Answer from the drawing. Dimensions are ordinates in mm from the lowest x, y and z of the part. A direction names the side the tool comes from. Give positions to 0.01 mm unless a question says otherwise; leave off trailing zeros. Write each loop counter-clockwise with the first axis right and the second up, starting at its lowest first coordinate (ties: lowest second). Pieces come first, ordered by that corner, then holes. Notation, with made-up numbers: M 26,18.25 L 66,18.25 A23 ccw 66,39.25 Z; hole C -26,57.25 d1. An arc over 180 degrees is marked long. Put each result on its own line as item: value.
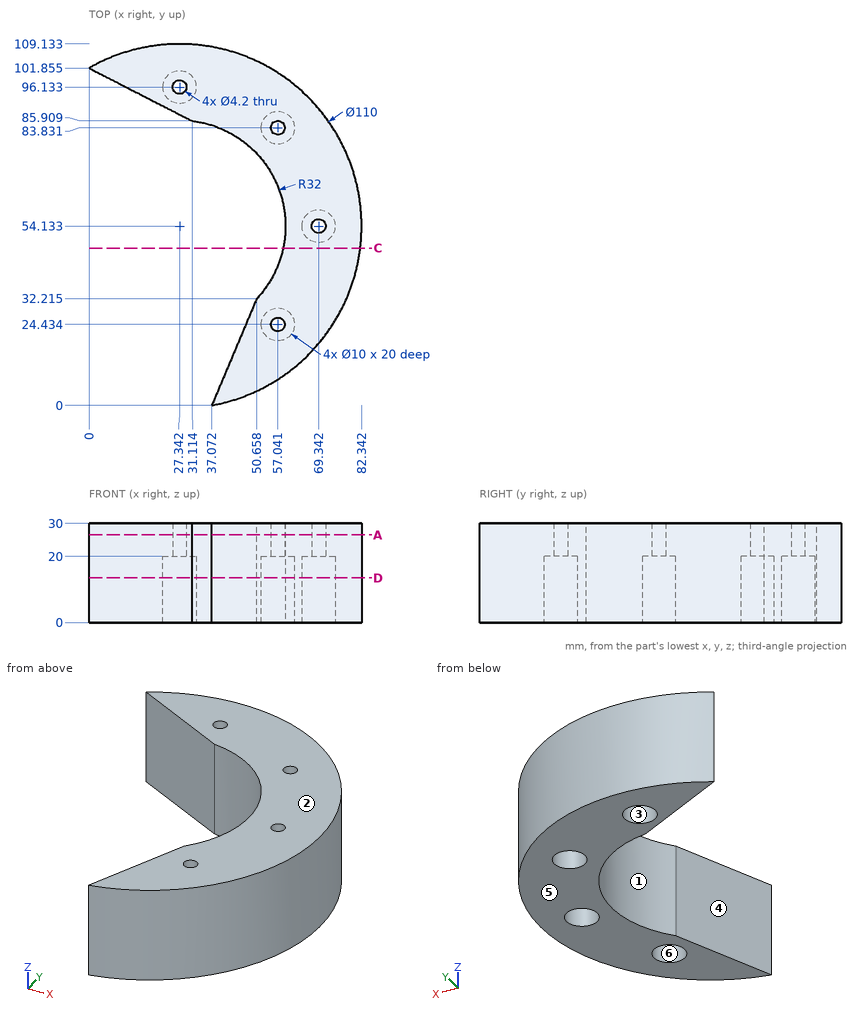
(1) Section A-A on z = 26.5 is taken. Determine the outline of the cut face in (x, y) (1 decimal).
Result:
outline: M 0,101.9 L 31.1,85.9 A32 cw 50.7,32.2 L 37.1,0 A55 ccw long Z; hole C 27.3,96.1 d4.2; hole C 57,24.4 d4.2; hole C 57,83.8 d4.2; hole C 69.3,54.1 d4.2
(2) Given pin 1 Ø8 at (x, y) = (71, 54) entering from -Z; pin 2 Ø2.5 at (x, y) = (69.34, 54.13) entering from +Z; pin 3 Ø3 at (x, z) = (60.5, 19.5) entering from -Y; pin 4 Ø2 at (y, z) = (90, 17) entering from -X, each flat-ended and moving along its own axis, determine where each tip first touches the part or whether it passes through.
Result:
pin 1: stops at z = 0
pin 2: passes through
pin 3: stops at y = 9.16
pin 4: stops at x = 21.18
(3) For a pull along X with two mould halves and no side action, classify the marked faces 1, 2 and 3 as +X half, -X half, draft (parallel to the pull), parting line (faces both ways), or undercut.
Result:
face 1: -X half
face 2: draft
face 3: undercut
(4) Which of the six approach directions +Z, -Z, +X, -X, +Y, -Y give full straight-line access (tool end or side, diameter ignored) to the marked faces 4, 5 and 6?
Result:
face 4: +Z, -Z, -X
face 5: -Z, +X, -X, +Y, -Y
face 6: -Z
(5) Straight lines are drawn through the part: line 1 along Y through (x, z) = (53, 17.5) (1 decimal); line 2 along X through (y, z) = (98, 4) (1 decimal); line 3 along X through (y, z) = (87, 12.75) (1 decimal). For each, find the intervals that lie inside material, in ascending order. Write a range as from..to.
Result:
line 1: y = 5.5..21.5, 27.4..35, 73.3..80.9, 86.8..102.8
line 2: x = 7.5..22.7, 32..60.5
line 3: x = 29..53.2, 60.9..71.4
(6) Section D-D on z = 13.5 is taken. Determine the outline of the cut face in (x, y) (1 decimal).
Result:
outline: M 0,101.9 L 31.1,85.9 A32 cw 50.7,32.2 L 37.1,0 A55 ccw long Z; hole C 27.3,96.1 d10; hole C 57,24.4 d10; hole C 57,83.8 d10; hole C 69.3,54.1 d10
(7) Section C-C on y = 47.5 is taken. Determine the outline of the cut face in (x, z), and give its area (3 significant figures).
Result:
outline: M 58.65,0 L 81.94,0 L 81.94,30 L 58.65,30 Z
area: 699 mm²
